from build123d import *

# Parameters (mm, degrees)
BOSS_EXTRUDE1_DEPTH = 30
SKETCH2_R           = 5
CUT_EXTRUDE1_DEPTH  = 114.247516529
CHAMFER1_SIZE       = 5
FILLET1_R           = 5


# Read off the part's stored shape, not the designer's step: Ø8.0mm Dowel Hole1
with BuildPart() as part:
    # Sketch1 → Boss-Extrude1 (new body)
    with BuildSketch(Plane(origin=(0, 0, 0), x_dir=(1, 0, 0), z_dir=(0, 1, 0))):
        with BuildLine():
            Line((-75, 30), (75, 30))
            ThreePointArc((75, 30), (105, 0), (75, -30))
            Line((75, -30), (-75, -30))
            ThreePointArc((-75, -30), (-105, 0), (-75, 30))
        make_face()
    extrude(amount=BOSS_EXTRUDE1_DEPTH)

    # Sketch2 → Cut-Extrude1 (cut, through all)
    with BuildSketch(Plane(origin=(0, 30, 0), x_dir=(1, 0, 0), z_dir=(0, 1, 0))):
        with Locations(Location((75, 0, 0), (0, 0, 270))):
            Circle(SKETCH2_R)
    extrude(amount=-CUT_EXTRUDE1_DEPTH, mode=Mode.SUBTRACT)

    # Chamfer1
    chamfer1_edges = [part.edges().sort_by_distance(p)[0] for p in [
        (105, 30, 0),
        (0, 30, -30),
        (-105, 30, 0),
        (0, 0, -30),
        (105, 0, 0),
        (0, 0, 30),
        (-105, 0, 0),
        (0, 30, 30),
    ]]
    chamfer(chamfer1_edges, length=CHAMFER1_SIZE)

    # Fillet1
    fillet1_edges = [part.edges().sort_by_distance(p)[0] for p in [
        (0, 25, 30),
        (0, 5, 30),
        (0, 0, -25),
        (-100, 0, 0),
        (100, 0, 0),
        (0, 0, 25),
        (105, 25, 0),
        (105, 5, 0),
        (-105, 25, 0),
        (-105, 5, 0),
        (0, 25, -30),
        (0, 5, -30),
        (0, 30, -25),
        (-100, 30, 0),
        (100, 30, 0),
        (0, 30, 25),
    ]]
    fillet(fillet1_edges, radius=FILLET1_R)

    # Ø8.0mm Dowel Hole1 outline → Ø8.0mm Dowel Hole1 (revolve, cut)
    with BuildSketch(Plane(origin=(-75, 0, 0), x_dir=(1, 0, 0), z_dir=(0, 0, 1))):
        Polygon((0, 30), (0, 17.596557524), (4, 20), (4, 30), align=None)
        Polygon((4, 10), (0, 12.403442476), (0, 0), (4, 0), align=None)
    revolve(axis=Axis((-75, 0, 0), (0, 1, 0)), mode=Mode.SUBTRACT)


solid = part.part
The listing builds one solid part. Answer for the finished solid, in the listing's coordinates (mm). A direction names the side the tool comes from. Give positions to 0.01 mm unless a question says otherwise; leave off trailing zeros. Write each loop counter-clockwise with the first axis right and the second up, starting at its lowest first coordinate (ties: lowest second). Pieces come first, ordered by that corner, then holes. Notation, with made-up numbers: (-2.75, -21.75) - (39.25, -21.75) arc R18 ccw to (39.25, 6.25) - close; hole circle Ø5 at (-11.75, 76.25). An arc over 180 degrees is marked (long way). One line per question, with ' | ' between items. Start each with the question number.
1. Determine the mould class of faces 1 (the face through (1.05, 29.61, -24.87)), 2 (the face through (-1.05, 24.82, 29.63)), 3 (the face through (-79, 5, 0)) for opening direction Z: +Z half, -Z half, draft (parallel to the pull), parting line (faces both ways), or undercut.
2. Straight lines are drawn through the part: line 1 (Z direction, x = -75, y = 23.25); line 2 (X direction, y = 7.5, z = 0); line 3 (X direction, y = 14.25, z = 0). For each, find the intervals that lie inside material, in ascending order.
3. For faces 4 (the face through (-101.789, 1.795, 0.589)), 5 (the face through (-79, 25, 0)), determine the directions among +Z, -Z, +X, -X, +Y, -Y from which every point of the face is accessible in a straight line to the end or side of a thin tool.
4. Given P1, Ø4, axis at y = 26.5, z = 20.5, coming from the -X side; P2, Ø2, axis at y = 7.5, z = -5.5, coming from the +X side; P3, Ø6.5, axis at x = -75, z = 0, coming from the +Y side, each flat-ended and moving along its own axis, determine where each tip first touches the part or whether it passes through.
5. Section A-A, the plane x = 2 is taken. Determine the outline of the cut face in (y, z), then the cut area to 3 significant figures.
Result:
1) face 1: -Z half | face 2: +Z half | face 3: undercut
2) line 1: z = -29.99 to -4, 4 to 29.99 | line 2: x = -105 to -79, -71 to 70, 80 to 105 | line 3: x = -105 to 70, 80 to 105
3) face 4: -X, -Y | face 5: +Y
4) P1: stops at x = -97.52 | P2: stops at x = 104.66 | P3: stops at y = 19.55
5) outline: (0, -22.93) arc R5 ccw to (1.46, -26.46) - (3.54, -28.54) arc R5 ccw to (7.07, -30) - (22.93, -30) arc R5 ccw to (26.46, -28.54) - (28.54, -26.46) arc R5 ccw to (30, -22.93) - (30, 22.93) arc R5 ccw to (28.54, 26.46) - (26.46, 28.54) arc R5 ccw to (22.93, 30) - (7.07, 30) arc R5 ccw to (3.54, 28.54) - (1.46, 26.46) arc R5 ccw to (0, 22.93) - close | area: 1,750 mm2
